Part model, mm, in its own coordinate system. Give positions to 0.01 mm unless a question says otherwise; leave off trailing zeros.
1. Probe line 1 (X direction, y = -7.75, z = 297); line 2 (Y direction, x = -15, z = 322); line 3 (X direction, y = -2.5, z = 398). List the from-to ranges inside material, lowest first.
2. Drop flat-ended pins along their axis: pin 1 Ø0.8 at (x, z) = (-14, 132) entering from -Y; pin 2 Ø3 at (y, z) = (-1, 225) entering from -X; pin 3 Ø1 at (y, z) = (3.5, 236.5) entering from +X. Give the stop position or say it passes through.
3. Slice it at A-A on z = 154. Give the number of separate pieces and of enclosed holes in the cut face, and give its area (3 significant figures).
from build123d import *

# Parameters (mm, degrees)
F0_R     = 2.1
F1_DEPTH = 465


with BuildPart() as f1:
    # F0 (on Top) → F1 (new body)
    with BuildSketch(Plane.XY):
        with BuildLine():
            Line((-5.398544, -10.060897), (-1.538544, -10.060897))
            Line((-1.538544, -10.060897), (1.461456, -10.060897))
            Line((1.461456, -10.060897), (5.321456, -10.060897))
            Line((5.321456, -10.060897), (7.121456, -8.260897))
            Line((7.121456, -8.260897), (4.462116, -8.260897))
            Line((4.462116, -8.260897), (4.462116, -6.620897))
            Line((4.462116, -6.620897), (7.121456, -3.961557))
            Line((7.121456, -3.961557), (9.711456, -3.961557))
            Line((9.711456, -3.961557), (9.961456, -3.711557))
            Line((9.961456, -3.711557), (10.211456, -3.961557))
            Line((10.211456, -3.961557), (12.801456, -3.961557))
            Line((12.801456, -3.961557), (15.460796, -6.620897))
            Line((15.460796, -6.620897), (15.460796, -8.260897))
            Line((15.460796, -8.260897), (12.801456, -8.260897))
            Line((12.801456, -8.260897), (14.601456, -10.060897))
            Line((14.601456, -10.060897), (18.461456, -10.060897))
            ThreePointArc((18.461456, -10.060897), (19.522116, -9.621557), (19.961456, -8.560897))
            Line((19.961456, -8.560897), (19.961456, -4.700897))
            Line((19.961456, -4.700897), (18.161456, -2.900897))
            Line((18.161456, -2.900897), (18.161456, -5.560237))
            Line((18.161456, -5.560237), (16.521456, -5.560237))
            Line((16.521456, -5.560237), (13.862116, -2.900897))
            Line((13.862116, -2.900897), (13.862116, -0.310897))
            Line((13.862116, -0.310897), (13.612116, -0.060897))
            Line((13.612116, -0.060897), (13.862116, 0.189103))
            Line((13.862116, 0.189103), (13.862116, 2.779103))
            Line((13.862116, 2.779103), (16.521456, 5.438443))
            Line((16.521456, 5.438443), (18.161456, 5.438443))
            Line((18.161456, 5.438443), (18.161456, 2.779103))
            Line((18.161456, 2.779103), (19.961456, 4.579103))
            Line((19.961456, 4.579103), (19.961456, 8.439103))
            ThreePointArc((19.961456, 8.439103), (19.522116, 9.499763), (18.461456, 9.939103))
            Line((18.461456, 9.939103), (14.601456, 9.939103))
            Line((14.601456, 9.939103), (12.801456, 8.139103))
            Line((12.801456, 8.139103), (15.460796, 8.139103))
            Line((15.460796, 8.139103), (15.460796, 6.499103))
            Line((15.460796, 6.499103), (12.801456, 3.839763))
            Line((12.801456, 3.839763), (10.211456, 3.839763))
            Line((10.211456, 3.839763), (9.961456, 3.589763))
            Line((9.961456, 3.589763), (9.711456, 3.839763))
            Line((9.711456, 3.839763), (7.121456, 3.839763))
            Line((7.121456, 3.839763), (4.462116, 6.499103))
            Line((4.462116, 6.499103), (4.462116, 8.139103))
            Line((4.462116, 8.139103), (7.121456, 8.139103))
            Line((7.121456, 8.139103), (5.321456, 9.939103))
            Line((5.321456, 9.939103), (1.461456, 9.939103))
            Line((1.461456, 9.939103), (-1.538544, 9.939103))
            Line((-1.538544, 9.939103), (-5.398544, 9.939103))
            Line((-5.398544, 9.939103), (-7.198544, 8.139103))
            Line((-7.198544, 8.139103), (-4.539204, 8.139103))
            Line((-4.539204, 8.139103), (-4.539204, 6.499103))
            Line((-4.539204, 6.499103), (-7.198544, 3.839763))
            Line((-7.198544, 3.839763), (-9.788544, 3.839763))
            Line((-9.788544, 3.839763), (-10.038544, 3.589763))
            Line((-10.038544, 3.589763), (-10.288544, 3.839763))
            Line((-10.288544, 3.839763), (-12.878544, 3.839763))
            Line((-12.878544, 3.839763), (-15.537884, 6.499103))
            Line((-15.537884, 6.499103), (-15.537884, 8.139103))
            Line((-15.537884, 8.139103), (-12.878544, 8.139103))
            Line((-12.878544, 8.139103), (-14.678544, 9.939103))
            Line((-14.678544, 9.939103), (-18.538544, 9.939103))
            ThreePointArc((-18.538544, 9.939103), (-19.599204, 9.499763), (-20.038544, 8.439103))
            Line((-20.038544, 8.439103), (-20.038544, 4.579103))
            Line((-20.038544, 4.579103), (-18.238544, 2.779103))
            Line((-18.238544, 2.779103), (-18.238544, 5.438443))
            Line((-18.238544, 5.438443), (-16.598544, 5.438443))
            Line((-16.598544, 5.438443), (-13.939204, 2.779103))
            Line((-13.939204, 2.779103), (-13.939204, 0.189103))
            Line((-13.939204, 0.189103), (-13.689204, -0.060897))
            Line((-13.689204, -0.060897), (-13.939204, -0.310897))
            Line((-13.939204, -0.310897), (-13.939204, -2.900897))
            Line((-13.939204, -2.900897), (-16.598544, -5.560237))
            Line((-16.598544, -5.560237), (-18.238544, -5.560237))
            Line((-18.238544, -5.560237), (-18.238544, -2.900897))
            Line((-18.238544, -2.900897), (-20.038544, -4.700897))
            Line((-20.038544, -4.700897), (-20.038544, -8.560897))
            ThreePointArc((-20.038544, -8.560897), (-19.599204, -9.621557), (-18.538544, -10.060897))
            Line((-18.538544, -10.060897), (-14.678544, -10.060897))
            Line((-14.678544, -10.060897), (-12.878544, -8.260897))
            Line((-12.878544, -8.260897), (-15.537884, -8.260897))
            Line((-15.537884, -8.260897), (-15.537884, -6.620897))
            Line((-15.537884, -6.620897), (-12.878544, -3.961557))
            Line((-12.878544, -3.961557), (-10.288544, -3.961557))
            Line((-10.288544, -3.961557), (-10.038544, -3.711557))
            Line((-10.038544, -3.711557), (-9.788544, -3.961557))
            Line((-9.788544, -3.961557), (-7.198544, -3.961557))
            Line((-7.198544, -3.961557), (-4.539204, -6.620897))
            Line((-4.539204, -6.620897), (-4.539204, -8.260897))
            Line((-4.539204, -8.260897), (-7.198544, -8.260897))
            Line((-7.198544, -8.260897), (-5.398544, -10.060897))
        make_face()
        Polygon((-16.607884, -7.690897), (-16.607884, -8.260897), (-18.238544, -8.260897), (-18.238544, -6.630237), (-17.668544, -6.630237), align=None, mode=Mode.SUBTRACT)
        Polygon((17.591456, -6.630237), (18.161456, -6.630237), (18.161456, -8.260897), (16.530796, -8.260897), (16.530796, -7.690897), align=None, mode=Mode.SUBTRACT)
        with Locations((-10.038544, -0.060897)):
            Circle(F0_R, mode=Mode.SUBTRACT)
        Polygon((-17.668544, 6.508443), (-18.238544, 6.508443), (-18.238544, 8.139103), (-16.607884, 8.139103), (-16.607884, 7.569103), align=None, mode=Mode.SUBTRACT)
        Polygon((-6.137884, 2.779103), (-3.478544, 5.438443), (-3.039204, 5.877783), (-3.039204, 8.139103), (2.962116, 8.139103), (2.962116, 5.877783), (3.401456, 5.438443), (6.060796, 2.779103), (6.060796, 0.189103), (6.310796, -0.060897), (6.060796, -0.310897), (6.060796, -2.900897), (3.401456, -5.560237), (2.962116, -5.999577), (2.962116, -8.260897), (-3.039204, -8.260897), (-3.039204, -5.999577), (-3.478544, -5.560237), (-6.137884, -2.900897), (-6.137884, -0.310897), (-6.387884, -0.060897), (-6.137884, 0.189103), align=None, mode=Mode.SUBTRACT)
        with Locations((9.961456, -0.060897)):
            Circle(F0_R, mode=Mode.SUBTRACT)
        Polygon((18.161456, 8.139103), (18.161456, 6.508443), (17.591456, 6.508443), (16.530796, 7.569103), (16.530796, 8.139103), align=None, mode=Mode.SUBTRACT)
    extrude(amount=F1_DEPTH)


solid = f1.part
Data:
1. line 1: x = -20.04 to -18.24, -16.61 to -15.54, -4.54 to -3.04, 2.96 to 4.46, 15.46 to 16.53, 18.16 to 19.96
1. line 2: y = -10.06 to -8.26, -6.08 to -3.96, 3.84 to 5.96, 8.14 to 9.94
1. line 3: x = -13.94 to -6.14, 6.06 to 13.86
2. pin 1: stops at y = -9.78
2. pin 2: stops at x = -13.94
2. pin 3: stops at x = 19.38
3. separate pieces: 1
3. enclosed holes: 7
3. area: 287 mm2
